from build123d import *

# Parameters (mm, degrees)
MODEL_R                 = 1.5
SALIENTE_EXTRUIR1_DEPTH = 3


with BuildPart() as part:
    # Model → Saliente-Extruir1 (new body)
    with BuildSketch(Plane.XY):
        with BuildLine():
            Line((256.429131311, 237.742243614), (346.429131311, 237.742243614))
            ThreePointArc((346.429131311, 237.742243614), (349.611111826, 236.424224129), (350.929131311, 233.242243614))
            Line((350.929131311, 233.242243614), (350.929131311, 215.242243614))
            ThreePointArc((350.929131311, 215.242243614), (349.611111826, 212.060263099), (346.429131311, 210.742243614))
            Line((346.429131311, 210.742243614), (256.429131311, 210.742243614))
            ThreePointArc((256.429131311, 210.742243614), (253.247150795, 212.060263099), (251.929131311, 215.242243614))
            Line((251.929131311, 215.242243614), (251.929131311, 233.242243614))
            ThreePointArc((251.929131311, 233.242243614), (253.247150795, 236.424224129), (256.429131311, 237.742243614))
        make_face()
        with Locations((310.429131311, 233.242243614)):
            Circle(MODEL_R, mode=Mode.SUBTRACT)
        with Locations((292.429131311, 233.242243614)):
            Circle(MODEL_R, mode=Mode.SUBTRACT)
        with Locations((301.429131311, 233.242243614)):
            Circle(MODEL_R, mode=Mode.SUBTRACT)
        with Locations((337.429131311, 215.242243614)):
            Circle(MODEL_R, mode=Mode.SUBTRACT)
        with Locations((319.429131311, 215.242243614)):
            Circle(MODEL_R, mode=Mode.SUBTRACT)
        with Locations((328.429131311, 215.242243614)):
            Circle(MODEL_R, mode=Mode.SUBTRACT)
        with Locations((310.429131311, 215.242243614)):
            Circle(MODEL_R, mode=Mode.SUBTRACT)
        with Locations((292.429131311, 215.242243614)):
            Circle(MODEL_R, mode=Mode.SUBTRACT)
        with Locations((301.429131311, 215.242243614)):
            Circle(MODEL_R, mode=Mode.SUBTRACT)
        with Locations((274.429131311, 215.242243614)):
            Circle(MODEL_R, mode=Mode.SUBTRACT)
        with Locations((283.429131311, 215.242243614)):
            Circle(MODEL_R, mode=Mode.SUBTRACT)
        with Locations((265.429131311, 215.242243614)):
            Circle(MODEL_R, mode=Mode.SUBTRACT)
        with Locations((256.429131311, 215.242243614)):
            Circle(MODEL_R, mode=Mode.SUBTRACT)
        with Locations((346.429131311, 215.242243614)):
            Circle(MODEL_R, mode=Mode.SUBTRACT)
        with Locations((274.429131311, 233.242243614)):
            Circle(MODEL_R, mode=Mode.SUBTRACT)
        with Locations((265.429131311, 233.242243614)):
            Circle(MODEL_R, mode=Mode.SUBTRACT)
        with Locations((256.429131311, 233.242243614)):
            Circle(MODEL_R, mode=Mode.SUBTRACT)
        with Locations((283.429131311, 233.242243614)):
            Circle(MODEL_R, mode=Mode.SUBTRACT)
        with Locations((337.429131311, 233.242243614)):
            Circle(MODEL_R, mode=Mode.SUBTRACT)
        with Locations((319.429131311, 233.242243614)):
            Circle(MODEL_R, mode=Mode.SUBTRACT)
        with Locations((328.429131311, 233.242243614)):
            Circle(MODEL_R, mode=Mode.SUBTRACT)
        with Locations((346.429131311, 233.242243614)):
            Circle(MODEL_R, mode=Mode.SUBTRACT)
        with Locations((337.429131311, 224.242243614)):
            Circle(MODEL_R, mode=Mode.SUBTRACT)
        with Locations((319.429131311, 224.242243614)):
            Circle(MODEL_R, mode=Mode.SUBTRACT)
        with Locations((328.429131311, 224.242243614)):
            Circle(MODEL_R, mode=Mode.SUBTRACT)
        with Locations((310.429131311, 224.242243614)):
            Circle(MODEL_R, mode=Mode.SUBTRACT)
        with Locations((292.429131311, 224.242243614)):
            Circle(MODEL_R, mode=Mode.SUBTRACT)
        with Locations((301.429131311, 224.242243614)):
            Circle(MODEL_R, mode=Mode.SUBTRACT)
        with Locations((274.429131311, 224.242243614)):
            Circle(MODEL_R, mode=Mode.SUBTRACT)
        with Locations((283.429131311, 224.242243614)):
            Circle(MODEL_R, mode=Mode.SUBTRACT)
        with Locations((265.429131311, 224.242243614)):
            Circle(MODEL_R, mode=Mode.SUBTRACT)
        with Locations((256.429131311, 224.242243614)):
            Circle(MODEL_R, mode=Mode.SUBTRACT)
        with Locations((346.429131311, 224.242243614)):
            Circle(MODEL_R, mode=Mode.SUBTRACT)
    extrude(amount=SALIENTE_EXTRUIR1_DEPTH)


solid = part.part
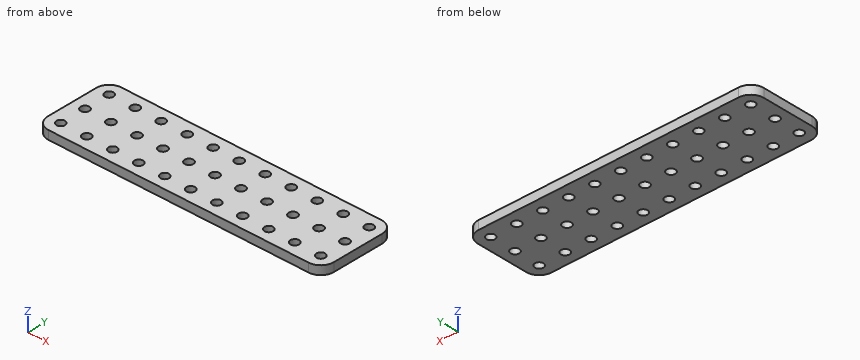
Here's how the part is built. I have some questions about the finished solid (model axes, mm). Coordinates: 2 decimals unless noted, no trailing zeros. Write each loop counter-clockwise with the first axis right and the second up, starting at its lowest first coordinate (ties: lowest second). Pieces come first, ordered by that corner, then holes.
Item 1: I want a section at B-B on z = 1.45. Count the separate pieces of the cut face and the enclosed holes in it, and give its area (3 significant figures).
Item 2: If I drill on line 1 (Y direction, x = 318.5, z = 2.45); line 2 (X direction, y = 212, z = 2.05), over which ranges is the centre line in solid material (lowest first)?
Item 3: I want a section at A-A on x = 310.5. Write out the boundary of the cut face in (y, z).
Item 4: I want a section at C-C on x = 275. Write out the boundary of the cut face in (y, z), and give its area (3 significant figures).
Findings below:
1. separate pieces: 1
1. enclosed holes: 33
1. area: 2,420 mm2
2. line 1: y = 210.74 to 214.06, 216.42 to 223.06, 225.42 to 232.06, 234.42 to 237.74
2. line 2: x = 253.31 to 349.55
3. outline: (210.74, 0) - (213.74, 0) - (213.74, 3) - (210.74, 3) - close; (216.74, 0) - (222.74, 0) - (222.74, 3) - (216.74, 3) - close; (225.74, 0) - (231.74, 0) - (231.74, 3) - (225.74, 3) - close; (234.74, 0) - (237.74, 0) - (237.74, 3) - (234.74, 3) - close
4. outline: (210.74, 0) - (213.86, 0) - (213.86, 3) - (210.74, 3) - close; (216.63, 0) - (222.86, 0) - (222.86, 3) - (216.63, 3) - close; (225.63, 0) - (231.86, 0) - (231.86, 3) - (225.63, 3) - close; (234.63, 0) - (237.74, 0) - (237.74, 3) - (234.63, 3) - close
4. area: 56.0 mm2
